Source: CAD feature listing. Evaluate the final solid. Frame: model axes, mm. Face numbers are marked on the shaded views. Coordinates: 2 decimals unless noted, no trailing zeros. Order: outer loops, then holes, each group sorted by start corner. A loop starts at its lowest first (then second) coordinate and runs counter-clockwise, first axis right, second up.
```python
from build123d import *

# Parameters (mm, degrees)
SKETCH_1_W          = 44
SKETCH_1_H          = 120
EXTRUDE_1_DEPTH     = 6
SKETCH_1_3_W        = 6
SKETCH_1_3_H        = 120
EXTRUDE_2_DEPTH     = 74
SKETCH_2_R          = 13
SKETCH_2_R_2        = 3
CUT_EXTRUDE_1_DEPTH = 7
SKETCH_3_R          = 2.5
CUT_EXTRUDE_2_DEPTH = 10
SKETCH_4_R          = 2
CUT_EXTRUDE_3_DEPTH = 20


with BuildPart() as part:
    # Sketch 1 → Extrude 1 (new body)
    with BuildSketch(Plane(origin=(0, 0, 0), x_dir=(1, 0, 0), z_dir=(0, 1, 0))):
        with Locations((-3, 0)):
            Rectangle(SKETCH_1_W, SKETCH_1_H)
    extrude(amount=EXTRUDE_1_DEPTH)

    # Sketch 1_3 → Extrude 2 (add)
    with BuildSketch(Plane(origin=(0, 0, 0), x_dir=(1, 0, 0), z_dir=(0, 1, 0))):
        with Locations((22, 0)):
            Rectangle(SKETCH_1_3_W, SKETCH_1_3_H)
    extrude(amount=EXTRUDE_2_DEPTH)

    # Sketch 2 → Cut-Extrude 1 (cut, through all)
    with BuildSketch(Plane.ZY.offset(-19)):
        with Locations((0, 49.5)):
            Circle(SKETCH_2_R)
        with Locations((-28, 49.5)):
            Circle(SKETCH_2_R_2)
        with Locations((28, 49.5)):
            Circle(SKETCH_2_R_2)
    extrude(amount=-CUT_EXTRUDE_1_DEPTH, mode=Mode.SUBTRACT)

    # Sketch 3 → Cut-Extrude 2 (cut)
    with BuildSketch(Plane(origin=(0, 6, 0), x_dir=(1, 0, 0), z_dir=(0, 1, 0))):
        with Locations((-18, 40)):
            Circle(SKETCH_3_R)
        with Locations((12, 40)):
            Circle(SKETCH_3_R)
        with Locations((-18, -40)):
            Circle(SKETCH_3_R)
        with Locations((12, -40)):
            Circle(SKETCH_3_R)
    extrude(amount=-CUT_EXTRUDE_2_DEPTH, mode=Mode.SUBTRACT)

    # Sketch 4 → Cut-Extrude 3 (cut)
    with BuildSketch(Plane(origin=(0, 0, -60), x_dir=(-1, 0, 0), z_dir=(0, 0, -1))):
        with Locations((-22, 17)):
            Circle(SKETCH_4_R)
        with Locations((-22, 57)):
            Circle(SKETCH_4_R)
    cut_extrude_3 = extrude(amount=-CUT_EXTRUDE_3_DEPTH, mode=Mode.SUBTRACT)

    # Mirror 1: Cut-Extrude 3 across plane
    add(cut_extrude_3.mirror(Plane(origin=(0, 0, 0), x_dir=(1, 0, 0), z_dir=(0, 0, -1))), mode=Mode.SUBTRACT)


solid = part.part
```
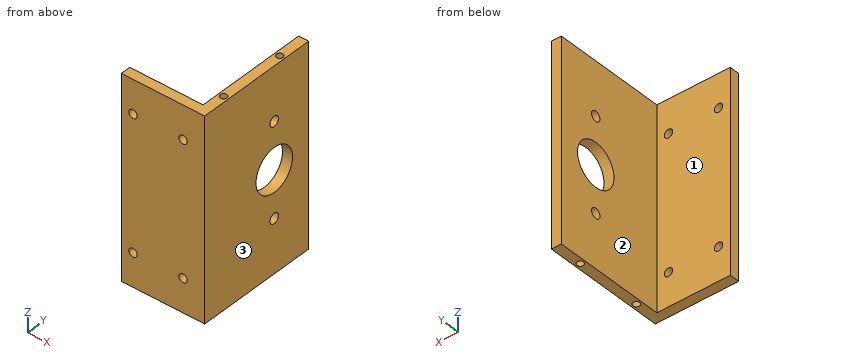
1. Ray query, line 1 (Y direction, x = 22, z = -53); line 2 (X direction, y = 3, z = -40); line 3 (Y direction, x = -17.5, z = 16.5). Return the intervals inside material, ascending.
Findings:
line 1: y = 0 to 15, 19 to 55, 59 to 74
line 2: x = -25 to -20.5, -15.5 to 9.5, 14.5 to 25
line 3: y = 0 to 6
2. Section query B-B on y = 49.5. Return loops of the section in (x, z), plus the area to 3 significant figures.
Findings:
outline: (19, -60) - (25, -60) - (25, -31) - (19, -31) - close; (19, -25) - (25, -25) - (25, -13) - (19, -13) - close; (19, 13) - (25, 13) - (25, 25) - (19, 25) - close; (19, 31) - (25, 31) - (25, 60) - (19, 60) - close
area: 492 mm2
3. Section query A-A on x = -18. Return loops of the section in (y, z), plus the area to 3 significant figures.
Findings:
outline: (0, -60) - (6, -60) - (6, -42.5) - (0, -42.5) - close; (0, -37.5) - (6, -37.5) - (6, 37.5) - (0, 37.5) - close; (0, 42.5) - (6, 42.5) - (6, 60) - (0, 60) - close
area: 660 mm2
4. Pin query (flat end, axial travel): P1, Ø8, axis at x = 12, z = 40, coming from the +Y side; P2, Ø3, axis at x = 22, y = 17, coming from the -Z side; P3, Ø1.2, axis at x = 22, y = 56.5, coming from the +Z side. Return the tip coordinate at first contact, or that it passes through.
Findings:
P1: stops at y = 6
P2: stops at z = -40
P3: stops at z = 40
5. Draft query along X for the marked faces 1, 2 and 3. Return one class per face: released by +X, released by -X, zero draft, split by the parting line, or undercut.
Findings:
face 1: zero draft
face 2: released by -X
face 3: released by +X
6. Section query C-C on z = -28. Return loops of the section in (x, y), plus the area to 3 significant figures.
Findings:
outline: (-25, 0) - (25, 0) - (25, 46.5) - (19, 46.5) - (19, 6) - (-25, 6) - close; (19, 52.5) - (25, 52.5) - (25, 74) - (19, 74) - close
area: 672 mm2
7. Section query D-D on y = 17. Return loops of the section in (x, z), plus the area to 3 significant figures.
Findings:
outline: (19, -60) - (20, -60) - (20, -40) - (24, -40) - (24, -60) - (25, -60) - (25, 60) - (24, 60) - (24, 40) - (20, 40) - (20, 60) - (19, 60) - close
area: 560 mm2
